```python
from build123d import *

# Parameters (mm, degrees)
F1_DEPTH      = 12.5
F1_DEPTH_BACK = 12.5
F4_D          = 6
F4_ON_F3_D    = 6


with BuildPart() as f1:
    # F0 (on Front) → F1 (new body, two sides)
    with BuildSketch(Plane.XZ) as f1_sk:
        with BuildLine():
            Line((5, 85), (0, 85))
            Line((0, 85), (0, 7))
            ThreePointArc((0, 7), (2.0502525317, 2.0502525317), (7, 0))
            Line((7, 0), (215, 0))
            Line((215, 0), (215, 5))
            Line((215, 5), (7, 5))
            ThreePointArc((7, 5), (5.5857864376, 5.5857864376), (5, 7))
            Line((5, 7), (5, 85))
        make_face()
    extrude(amount=F1_DEPTH)
    extrude(f1_sk.sketch, amount=-F1_DEPTH_BACK)

    # F4 (through all)
    with Locations(Plane(origin=(0, 0, 0), x_dir=(1, 0, 0), z_dir=(0, 0, -1))):
        with Locations((200, 0), (135, 0), (40, 0)):
            Hole(F4_D / 2)

    # F4 on F3 (through all)
    with Locations(Plane(origin=(0, 0, 0), x_dir=(0, -1, 0), z_dir=(-1, 0, 0))):
        with Locations((0, 40), (0, 71)):
            Hole(F4_ON_F3_D / 2)


solid = f1.part
```
Geometry: final body of the model. Coordinates: model frame, mm. A direction names the side the tool comes from. Coordinates: 2 decimals unless noted, no trailing zeros. Order: outer loops, then holes, each group sorted by start corner. A loop starts at its lowest first (then second) coordinate and runs counter-clockwise, first axis right, second up. Notation, with made-up numbers: M 52.25,-21.75 L 92.25,-21.75 A30 cw 92.25,8.25 Z; hole C 58,30 d2. An arc over 180 degrees is marked long. Answer in a Markdown table with one row per item. Add a question column.
Q1. Section query A-A on y = 0. Return the cut outline in (x, z).
Q2. Contact query for flat-ended pins moving along their axis: P1, Ø2, axis at y = -7.5, z = 26, coming from the +X side; P2, Ø7, axis at x = 135, y = 0, coming from the -Z side; P3, Ø12, axis at x = 41.5, y = -10, coming from the +Z side. Output: stop coordinate, or through.
Q3. Section query C-C on z = 40. Return the cut outline in (x, y), and give its area (3 significant figures).
Q4. Line query: L1, parallel to Y at x = 40, z = 2; L2, parallel to X at y = -7.5, z = 21.5. Output: solid intervals per line, ascending.
Q5. Section query D-D on x = 153.5. Return the cut outline in (y, z).
Q6. Section query B-B on x = 40. Return the cut outline in (y, z).
Q7. Mould query, pull axis Y, two halves, no side actions, for faces 1 (the flat face through (75, 12.5, 2)), 2 (the flat face through (112, 0, 5)), 3 (the cylindrical face through (2.53, -0.65, 68.07)). Classes: released by +Y, released by -Y, zero draft, split by the parting line, or undercut.
Q8. Reachability of faces 4 (the flat face through (5, 0, 45)), 5 (the cylindrical face through (2, -0.2, 2.1)) from +Z, -Z, +X, -X, +Y, -Y: full face, straight path, thin tool, end or side. Return the list, or none.
Completed:
| question | item | result |
|---|---|---|
| 1 | outline | M 0,7 A7 ccw 7,0 L 37,0 L 37,5 L 7,5 A2 cw 5,7 L 5,37 L 0,37 Z; M 0,43 L 5,43 L 5,68 L 0,68 Z; M 0,74 L 5,74 L 5,85 L 0,85 Z; M 43,0 L 132,0 L 132,5 L 43,5 Z; M 138,0 L 197,0 L 197,5 L 138,5 Z; M 203,0 L 215,0 L 215,5 L 203,5 Z |
| 2 | P1 | stops at x = 5 |
| 2 | P2 | stops at z = 0 |
| 2 | P3 | stops at z = 5 |
| 3 | outline | M 0,-12.5 L 5,-12.5 L 5,-3 L 0,-3 Z; M 0,3 L 5,3 L 5,12.5 L 0,12.5 Z |
| 3 | area | 95.0 mm2 |
| 4 | L1 | y = -12.5 to -3, 3 to 12.5 |
| 4 | L2 | x = 0 to 5 |
| 5 | outline | M -12.5,0 L 12.5,0 L 12.5,5 L -12.5,5 Z |
| 6 | outline | M -12.5,0 L -3,0 L -3,5 L -12.5,5 Z; M 3,0 L 12.5,0 L 12.5,5 L 3,5 Z |
| 7 | face 1 | released by +Y |
| 7 | face 2 | zero draft |
| 7 | face 3 | undercut |
| 8 | face 4 | +Z, +X, +Y, -Y |
| 8 | face 5 | -Z, -X, +Y, -Y |
